from build123d import *

# Parameters (mm, degrees)
F1_DEPTH = 2.5


with BuildPart() as f1:
    # F0 (on Top) → F1 (new body)
    with BuildSketch(Plane.XY):
        with BuildLine():
            Line((51.910336, 20.642742), (-58.089664, 20.642742))
            ThreePointArc((-58.089664, 20.642742), (-61.625198, 19.178275), (-63.089664, 15.642742))
            Line((-63.089664, 15.642742), (-63.089664, -14.357258))
            ThreePointArc((-63.089664, -14.357258), (-61.625198, -17.892792), (-58.089664, -19.357258))
            Line((-58.089664, -19.357258), (51.910336, -19.357258))
            ThreePointArc((51.910336, -19.357258), (55.44587, -17.892792), (56.910336, -14.357258))
            Line((56.910336, -14.357258), (56.910336, 15.642742))
            ThreePointArc((56.910336, 15.642742), (55.44587, 19.178275), (51.910336, 20.642742))
        make_face()
        with BuildLine():
            Line((50.540434, -14.357258), (-56.719762, -14.357258))
            ThreePointArc((-56.719762, -14.357258), (-57.688429, -13.956023), (-58.089664, -12.987356))
            Line((-58.089664, -12.987356), (-58.089664, -11.727161))
            ThreePointArc((-58.089664, -11.727161), (-57.688429, -10.758493), (-56.719762, -10.357258))
            Line((-56.719762, -10.357258), (50.540434, -10.357258))
            ThreePointArc((50.540434, -10.357258), (51.509101, -10.758493), (51.910336, -11.727161))
            Line((51.910336, -11.727161), (51.910336, -12.987356))
            ThreePointArc((51.910336, -12.987356), (51.509101, -13.956023), (50.540434, -14.357258))
        make_face(mode=Mode.SUBTRACT)
        with BuildLine():
            ThreePointArc((-58.089664, 14.272839), (-57.688429, 15.241507), (-56.719762, 15.642742))
            Line((-56.719762, 15.642742), (50.540434, 15.642742))
            ThreePointArc((50.540434, 15.642742), (51.509101, 15.241507), (51.910336, 14.272839))
            Line((51.910336, 14.272839), (51.910336, 13.012644))
            ThreePointArc((51.910336, 13.012644), (51.509101, 12.043977), (50.540434, 11.642742))
            Line((50.540434, 11.642742), (-56.719762, 11.642742))
            ThreePointArc((-56.719762, 11.642742), (-57.688429, 12.043977), (-58.089664, 13.012644))
            Line((-58.089664, 13.012644), (-58.089664, 14.272839))
        make_face(mode=Mode.SUBTRACT)
    extrude(amount=F1_DEPTH)


solid = f1.part
Source: CAD feature listing. Evaluate the final solid. Frame: model axes, mm. A direction names the side the tool comes from. Give positions to 0.01 mm unless a question says otherwise; leave off trailing zeros. Write each loop counter-clockwise with the first axis right and the second up, starting at its lowest first coordinate (ties: lowest second). Pieces come first, ordered by that corner, then holes. Notation, with made-up numbers: M 68.25,63.25 L 75.25,63.25 A26 ccw 75.25,81.25 Z; hole C 84.25,30 d1. An arc over 180 degrees is marked long. Return JSON: item names as keys, results as strings. Group by question number.
1) Set-up query: faces 4 (the face through (-2, -14.357, 1)), 5 (the face through (-4, -19.357, 1)). Return all of +Z, -Z, +X, -X, +Y, -Y with unobstructed straight access to the full face (end or side cutting, diameter ignored); none if empty.
2) Ray query, L1, parallel to Y at x = 18, z = 0.85; L2, parallel to Y at x = -57, z = 2.3; L3, parallel to X at y = 18.5, z = 1.8. Return the intervals inside material, ascending.
3) Draft query along Y for faces 1 (the face through (-63.09, 1, 1)), 2 (the face through (55.41, -17.93, 1.23)), 3 (the face through (-2, 11.643, 1)). Return one class per face: released by +Y, released by -Y, zero draft, split by the parting line, or undercut.
4) Cut plane B-B, the plane z = 1.85. Output: boundary loops of the cut face in (x, y).
5) Cut plane A-A, the plane x = -31.5. Output: boundary loops of the cut face in (y, z).
Data:
{
 "1": {"face 4": "+Z, -Z", "face 5": "+Z, -Z, +X, -X, -Y"},
 "2": {"L1": "y = -19.36 to -14.36, -10.36 to 11.64, 15.64 to 20.64", "L2": "y = -19.36 to -14.33, -10.39 to 11.67, 15.61 to 20.64", "L3": "x = -62.19 to 56.01"},
 "3": {"face 1": "zero draft", "face 2": "released by -Y", "face 3": "undercut"},
 "4": {"outline": "M -63.09,-14.36 A5 ccw -58.09,-19.36 L 51.91,-19.36 A5 ccw 56.91,-14.36 L 56.91,15.64 A5 ccw 51.91,20.64 L -58.09,20.64 A5 ccw -63.09,15.64 Z; hole M -58.09,-12.99 A1.37 ccw -56.72,-14.36 L 50.54,-14.36 A1.37 ccw 51.91,-12.99 L 51.91,-11.73 A1.37 ccw 50.54,-10.36 L -56.72,-10.36 A1.37 ccw -58.09,-11.73 Z; hole M -58.09,13.01 A1.37 ccw -56.72,11.64 L 50.54,11.64 A1.37 ccw 51.91,13.01 L 51.91,14.27 A1.37 ccw 50.54,15.64 L -56.72,15.64 A1.37 ccw -58.09,14.27 Z"},
 "5": {"outline": "M -19.36,0 L -14.36,0 L -14.36,2.5 L -19.36,2.5 Z; M -10.36,0 L 11.64,0 L 11.64,2.5 L -10.36,2.5 Z; M 15.64,0 L 20.64,0 L 20.64,2.5 L 15.64,2.5 Z"}
}
